```python
from build123d import *

# Parameters (mm, degrees)
ESQUISSE1_W             = 197
ESQUISSE1_H             = 309
ESQUISSE1_R             = 1.7
ESQUISSE1_R_2           = 3
BOSS_EXTRU_1_DEPTH      = 3
ESQUISSE2_W             = 60
ESQUISSE2_H             = 234
ENL_V_MAT_EXTRU_1_DEPTH = 4
CONG_1_R                = 10


with BuildPart() as part:
    # Esquisse1 → Boss.-Extru.1 (new body)
    with BuildSketch(Plane.XY):
        Rectangle(ESQUISSE1_W, ESQUISSE1_H)
        with Locations((81.25, 121.5)):
            Circle(ESQUISSE1_R, mode=Mode.SUBTRACT)
        with Locations((64.5, 121.5)):
            Circle(ESQUISSE1_R_2, mode=Mode.SUBTRACT)
        with Locations((81.25, -121.5)):
            Circle(ESQUISSE1_R, mode=Mode.SUBTRACT)
        with Locations((64.5, -121.5)):
            Circle(ESQUISSE1_R_2, mode=Mode.SUBTRACT)
        with Locations((-81.25, -121.5)):
            Circle(ESQUISSE1_R, mode=Mode.SUBTRACT)
        with Locations((-64.5, -121.5)):
            Circle(ESQUISSE1_R_2, mode=Mode.SUBTRACT)
        with Locations((-81.25, 121.5)):
            Circle(ESQUISSE1_R, mode=Mode.SUBTRACT)
        with Locations((-64.5, 121.5)):
            Circle(ESQUISSE1_R_2, mode=Mode.SUBTRACT)
    extrude(amount=BOSS_EXTRU_1_DEPTH)

    # Esquisse2 → Enlèv. mat.-Extru.1 (cut, through all)
    with BuildSketch(Plane.XY.offset(3)):
        with Locations((-68.5, -37.5)):
            Rectangle(ESQUISSE2_W, ESQUISSE2_H)
    extrude(amount=-ENL_V_MAT_EXTRU_1_DEPTH, mode=Mode.SUBTRACT)

    # Congé1
    cong_1_edges = [part.edges().sort_by_distance(p)[0] for p in [
        (-98.5, 79.5, 1.5),
        (-38.5, 79.5, 1.5),
    ]]
    fillet(cong_1_edges, radius=CONG_1_R)


solid = part.part
```
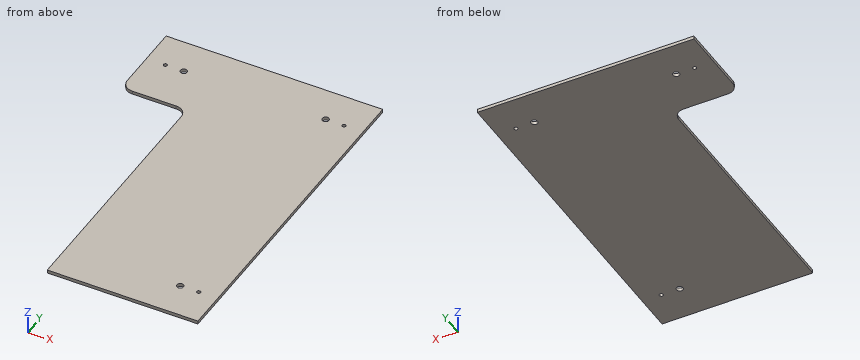
CAD build for the part. Positions are in the model's coordinates, mm. Give positions to 0.01 mm unless a question says otherwise; leave off trailing zeros. Write each loop counter-clockwise with the first axis right and the second up, starting at its lowest first coordinate (ties: lowest second). Pieces come first, ordered by that corner, then holes. Notation, with made-up numbers: (72.5, 31) -> (125.5, 31) arc R25 ccw to (125.5, 68) -> close; hole circle Ø5 at (33.25, 0). An arc over 180 degrees is marked (long way). Write each question's results on one line, items separated by ' | '.
1. Cut at C-C, the plane x = -64.5. Write the cut outline in (y, z), then the cut area to 3 significant figures.
Geometry check:
outline: (79.5, 0) -> (118.5, 0) -> (118.5, 3) -> (79.5, 3) -> close; (124.5, 0) -> (154.5, 0) -> (154.5, 3) -> (124.5, 3) -> close | area: 207 mm²
2. Cut at D-D, the plane y = -19. Write the cut outline in (x, z), then the cut area to 3 significant figures.
Geometry check:
outline: (-38.5, 0) -> (98.5, 0) -> (98.5, 3) -> (-38.5, 3) -> close | area: 411 mm²
3. Cut at A-A, the plane x = 64.5. Write the cut outline in (y, z).
Geometry check:
outline: (-154.5, 0) -> (-124.5, 0) -> (-124.5, 3) -> (-154.5, 3) -> close; (-118.5, 0) -> (118.5, 0) -> (118.5, 3) -> (-118.5, 3) -> close; (124.5, 0) -> (154.5, 0) -> (154.5, 3) -> (124.5, 3) -> close
4. Drop a flat-ended pin along its axis: P1, Ø1, axis at y = -102, z = 0.5, coming from the -X side. Give the stop position or say it passes through.
Geometry check:
P1: x = -38.5
5. Wall check: probe 1 along Y at (x, z) = (64.5, 1.2); probe 2 along Y at (x, z) = (81.25, 2); probe 3 along X at (y, z) = (-125, 0.6). Give the ranges that are in metal, low to high. Write a range as [from, to].
Geometry check:
probe 1: [-154.5, -124.5], [-118.5, 118.5], [124.5, 154.5] | probe 2: [-154.5, -123.2], [-119.8, 119.8], [123.2, 154.5] | probe 3: [-38.5, 98.5]
6. Cut at B-B, the plane z = 1.4. Write the cut outline in (x, y), then the cut area to 3 significant figures.
Geometry check:
outline: (-98.5, 89.5) arc R10 ccw to (-88.5, 79.5) -> (-48.5, 79.5) arc R10 cw to (-38.5, 69.5) -> (-38.5, -154.5) -> (98.5, -154.5) -> (98.5, 154.5) -> (-98.5, 154.5) -> close; hole circle Ø3.4 at (-81.25, 121.5); hole circle Ø6 at (-64.5, 121.5); hole circle Ø6 at (64.5, -121.5); hole circle Ø6 at (64.5, 121.5); hole circle Ø3.4 at (81.25, -121.5); hole circle Ø3.4 at (81.25, 121.5) | area: 46,700 mm²
